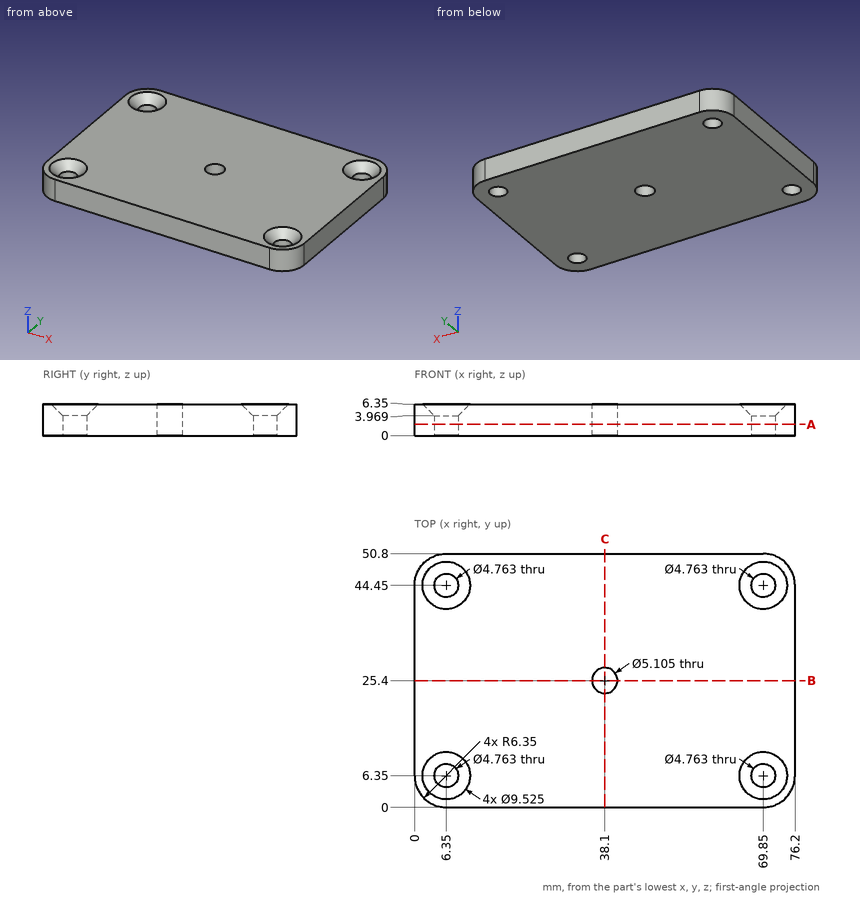
Geometry check sheet. Reference: drawing and pictorial views, mm from the part's lowest x, y, z. Give positions to 0.01 mm unless a question says otherwise; leave off trailing zeros. Order: outer loops, then holes, each group sorted by start corner. A loop starts at its lowest first (then second) coordinate and runs counter-clockwise, first axis right, second up. Notation, with made-up numbers: M -35,34.25 L -17,34.25 A19 cw -17,49.25 Z; hole C -25.75,-19.5 d6. An arc over 180 degrees is marked long. Answer as a JSON object with one key per item and string values. Group by question number.
1) Scan lines: line 1 along X through (y, z) = (8, 4.5); line 2 along Y through (x, z) = (6.35, 1.2); line 3 along X through (y, z) = (25.4, 3.75). Record each from-to range of solid material in increasing order. Write a range as [from, to].
2) Cross-section at A-A (z = 2.25). Give the number of separate pieces and of enclosed holes in the cut face, then the cut area to 3 significant figures.
3) Cross-section at B-B (y = 25.4). Enter the section's corners in (x, z).
4) Cross-section at C-C (x = 38.1). Enter the section's corners in (y, z).
Result sheet:
{
 "1": {"line 1": "x = [0, 3.95], [8.75, 67.45], [72.25, 76.2]", "line 2": "y = [0, 3.97], [8.73, 42.07], [46.83, 50.8]", "line 3": "x = [0, 35.55], [40.65, 76.2]"},
 "2": {"separate pieces": "1", "enclosed holes": "5", "area": "3,740 mm2"},
 "3": {"outline": "M 0,0 L 35.55,0 L 35.55,6.35 L 0,6.35 Z; M 40.65,0 L 76.2,0 L 76.2,6.35 L 40.65,6.35 Z"},
 "4": {"outline": "M 0,0 L 22.85,0 L 22.85,6.35 L 0,6.35 Z; M 27.95,0 L 50.8,0 L 50.8,6.35 L 27.95,6.35 Z"}
}
